Geometry: final body of the model. Coordinates: model frame, mm. A direction names the side the tool comes from. Coordinates: 2 decimals unless noted, no trailing zeros. Write each loop counter-clockwise with the first axis right and the second up, starting at its lowest first coordinate (ties: lowest second). Pieces come first, ordered by that corner, then holes. Notation, with made-up numbers: (66, 44.5) -> (83, 44.5) arc R13 ccw to (83, 65.5) -> close; hole circle Ø5 at (-22.75, -31). An arc over 180 degrees is marked (long way). Answer as a JSON object with one key per item and string values. Group by question number.
```python
from build123d import *

# Parameters (mm, degrees)
F0_R        = 1.5
F0_R_2      = 1.5885930288
F0_R_3      = 2.5
F1_DEPTH    = 2.5
F2_T1_DEPTH = 30.7168298797
F3_R        = 10


# Not quite as in the source:
# - a fillet or chamfer that OpenCascade refuses, or shapes differently, is made with other operations: its cross-section is extruded or revolved along the edge and cut away or added


with BuildPart() as f1:
    # F0 (on Front) → F1 (new body)
    with BuildSketch(Plane.XZ):
        with BuildLine():
            Line((-0.0187197208, 13.0832688883), (5.6909857328, 24.2902945465))
            ThreePointArc((5.6909857328, 24.2902945465), (-2.5187197208, 40), (-10.7284251743, 24.2902945465))
            Line((-10.7284251743, 24.2902945465), (-5.0187197208, 13.0832688883))
            Line((-5.0187197208, 13.0832688883), (-5.0187197208, -20))
            Line((-5.0187197208, -20), (-0.0187197208, -20))
            Line((-0.0187197208, -20), (-0.0187197208, 13.0832688883))
        make_face()
        with Locations((-2.5187197208, 6.5416344441)):
            Circle(F0_R, mode=Mode.SUBTRACT)
        with Locations((-2.5187197208, -6.5)):
            Circle(F0_R_2, mode=Mode.SUBTRACT)
        with Locations((-2.5187197208, 30)):
            Circle(F0_R_3, mode=Mode.SUBTRACT)
    extrude(amount=F1_DEPTH)

    # F2: chamfer of 5 on 1 edges, made by hand

    # F2_s2 → F2_t1 (cut)
    with BuildSketch(Plane.YZ.offset(-17.8771346606)):
        Polygon((2.5, -20), (-2.5, -15), (-2.5, -20), align=None)
    extrude(amount=F2_T1_DEPTH, mode=Mode.SUBTRACT)

    # F3
    f3_edges = [f1.edges().sort_by_distance(p)[0] for p in [
        (-0.01872, -1.25, 13.083269),
        (-5.01872, -1.25, 13.083269),
        (5.690986, -1.25, 24.290295),
        (-10.728425, -1.25, 24.290295),
    ]]
    fillet(f3_edges, radius=F3_R)


solid = f1.part
```
Item 1: Mould query, pull axis Z, two halves, no side actions, for faces 4 (the flat face through (-3, 0, 18)), 5 (the cylindrical face through (-5.303, -1.268, 13.049)), 6 (the cylindrical face through (-1.003, -1.232, -6.023)). Classes: +Z half, -Z half, draft (parallel to the pull), parting line (faces both ways), or undercut.
Item 2: Ray query, L1, parallel to Z at x = -3.25, y = -1.4; L2, parallel to X at y = -1.7, z = 29; L3, parallel to X at y = -0.55, z = -7. Return the intervals inside material, ascending. Write a range as [from, to].
Item 3: Contact query for flat-ended pins moving along their axis: pin 1 (8 mm diameter, centred on x = 2, z = -4.5, fed in from +Y); pin 2 (2.5 mm diameter, centred on x = -2.52, z = 6.54, fed in from -Y); pin 3 (0.8 mm diameter, centred on y = -2, z = -5.5, fed in from -X); pin 4 (1.5 mm diameter, centred on x = 1.5, y = -2, fed in from +Z). Output: stop coordinate, or through.
Item 4: Section D-D on z = 9.5. Output: boundary loops of the cut face in (x, y), then the cut area to 3 significant figures.
Item 5: Set-up query: faces 1 (the cylindrical face through (-2.844, -1.232, 5.077)), 2 (the flat face through (-0.019, -1, -4)), 3 (the flat face through (-5.019, -1, -3)). Return all of +Z, -Z, +X, -X, +Y, -Y with unobstructed straight access to the full face (end or side cutting, diameter ignored); none if empty.
Item 6: Section B-B on y = -1.9. Output: boundary loops of the cut face in (x, z).
Item 7: Section A-A on z = 30. Output: boundary loops of the cut face in (x, y).
Item 8: Section C-C on z = -6.5. Output: boundary loops of the cut face in (x, y), then the cut area to 3 significant figures.
Answer sheet:
{
 "1": {"face 4": "draft", "face 5": "-Z half", "face 6": "undercut"},
 "2": {"L1": "z = [-16.1, -7.91], [-5.09, 5.23], [7.85, 27.61], [32.39, 39.97]", "L2": "x = [-12.47, -4.81], [-0.23, 7.43]", "L3": "x = [-5.02, -4.03], [-1.01, -0.02]"},
 "3": {"pin 1": "stops at y = 0", "pin 2": "passes through", "pin 3": "stops at x = -5.02", "pin 4": "stops at z = 39.45"},
 "4": {"outline": "(-5.02, -2.5) -> (-0.02, -2.5) -> (-0.02, 0) -> (-5.02, 0) -> close", "area": "12.5 mm^2"},
 "5": {"face 1": "+Y, -Y", "face 2": "-Z, +X, +Y, -Y", "face 3": "-Z, -X, +Y, -Y"},
 "6": {"outline": "(-10.95, 24.62) arc R10 cw to (-10.47, 23.79) -> (-6.11, 15.22) arc R10 cw to (-5.02, 10.68) -> (-5.02, -15.6) -> (-0.02, -15.6) -> (-0.02, 10.68) arc R10 cw to (1.07, 15.22) -> (5.43, 23.79) arc R10 cw to (5.91, 24.62) arc R10 ccw (long way) to start; hole circle Ø5 at (-2.52, 30); hole circle Ø3.18 at (-2.52, -6.5); hole circle Ø3 at (-2.52, 6.54)"},
 "7": {"outline": "(-12.52, -2.5) -> (-5.02, -2.5) -> (-5.02, 0) -> (-12.52, 0) -> close; (-0.02, -2.5) -> (7.48, -2.5) -> (7.48, 0) -> (-0.02, 0) -> close"},
 "8": {"outline": "(-5.02, -2.5) -> (-4.11, -2.5) -> (-4.11, 0) -> (-5.02, 0) -> close; (-0.93, -2.5) -> (-0.02, -2.5) -> (-0.02, 0) -> (-0.93, 0) -> close", "area": "4.56 mm^2"}
}
